Part model, mm, in its own coordinate system. A direction names the side the tool comes from. Give positions to 0.01 mm unless a question says otherwise; leave off trailing zeros. Write each loop counter-clockwise with the first axis right and the second up, starting at its lowest first coordinate (ties: lowest second). Pieces come first, ordered by that corner, then holes.
```python
from build123d import *

# Parameters (mm, degrees)
CROQUIS1_W              = 50
CROQUIS1_H              = 25
SALIENTE_EXTRUIR1_DEPTH = 20
SALIENTE_EXTRUIR2_DEPTH = 25
SALIENTE_EXTRUIR3_DEPTH = 2
CROQUIS3_W              = 40
CROQUIS3_H              = 23
CORTAR_EXTRUIR1_DEPTH   = 20
CHAFL_N1_SIZE           = 5
CHAFL_N1_SIZE2          = 5.958767963


with BuildPart() as part:
    # Croquis1 → Saliente-Extruir1 (new body)
    with BuildSketch(Plane(origin=(0, 0, 0), x_dir=(1, 0, 0), z_dir=(0, 1, 0))):
        Rectangle(CROQUIS1_W, CROQUIS1_H)
    extrude(amount=SALIENTE_EXTRUIR1_DEPTH)

    # Croquis2 → Saliente-Extruir2 (add)
    with BuildSketch(Plane.XY.offset(12.5)):
        with BuildLine():
            ThreePointArc((25, 20), (3, 42), (-19, 20))
            Line((-19, 20), (-17, 20))
            ThreePointArc((-17, 20), (3, 40), (23, 20))
            Line((23, 20), (25, 20))
        make_face()
    extrude(amount=-SALIENTE_EXTRUIR2_DEPTH)

    # Croquis2<6> → Saliente-Extruir3 (add)
    with BuildSketch(Plane.XY.offset(12.5)):
        with BuildLine():
            ThreePointArc((23, 20), (3, 40), (-17, 20))
            Line((-17, 20), (23, 20))
        make_face()
    extrude(amount=-SALIENTE_EXTRUIR3_DEPTH)

    # Croquis3 → Cortar-Extruir1 (cut)
    with BuildSketch(Plane(origin=(0, 20, 0), x_dir=(1, 0, 0), z_dir=(0, 1, 0))):
        with Locations((3, 1)):
            Rectangle(CROQUIS3_W, CROQUIS3_H)
    extrude(amount=-CORTAR_EXTRUIR1_DEPTH, mode=Mode.SUBTRACT)

    # Chaflán1
    chafl_n1_edges = [part.edges().sort_by_distance(p)[0] for p in [
        (-25, 20, 0),
    ]]
    chafl_n1_side = [part.faces().sort_by_distance(p)[0] for p in [
        (-25, 10, 0),
    ]]
    chamfer(chafl_n1_edges, length=CHAFL_N1_SIZE, length2=CHAFL_N1_SIZE2, reference=chafl_n1_side[0])


solid = part.part
```
1) 3-axis set-ups, long thin cutter, end or side, ignore diameter. For faces 5 (the face through (-21.979, 17.535, 0.175)), 6 (the face through (-17, 10, -1)): which of +Z, -Z, +X, -X, +Y, -Y reach the whole face in a straight line?
Answers follow:
face 5: +Z, -Z, -X, +Y
face 6: -Z, -Y
2) Saw through at C-C, the plane y = 12.5. Write the cut outline in (x, z), then the cut area to 3 significant figures.
Answers follow:
outline: (-25, -12.5) - (-17, -12.5) - (-17, 10.5) - (23, 10.5) - (23, -12.5) - (25, -12.5) - (25, 12.5) - (-25, 12.5) - close
area: 330 mm2
3) Saw through at B-B, the plane x = 3. Write the cut outline in (y, z).
Answers follow:
outline: (0, 10.5) - (40, 10.5) - (40, -12.5) - (42, -12.5) - (42, 12.5) - (0, 12.5) - close
4) Pin check, flat tips, straight feed: pin 1 Ø10 at (x, z) = (-8, 10) entering from +Y; pin 2 Ø2 at (x, z) = (8.5, -9) entering from -Y; pin 3 Ø1.5 at (x, y) = (8, 22) entering from -Z. Stop position of each tip, or through.
Answers follow:
pin 1: stops at y = 41.17
pin 2: stops at y = 38.91
pin 3: stops at z = 10.5
5) Wall check: L1, parallel to X at y = 12, z = 10; L2, parallel to Z at x = 8, y = 34.5; L3, parallel to X at y = 37, z = 9.5. Give the ranges that are in metal, low to high.
Answers follow:
L1: x = -25 to -17, 23 to 25
L2: z = 10.5 to 12.5
L3: x = -10.96 to -7.54, 13.54 to 16.96
6) Saw through at D-D, the plane x = -7.5. Write the cut outline in (y, z).
Answers follow:
outline: (0, 10.5) - (37.02, 10.5) - (37.02, -12.5) - (39.33, -12.5) - (39.33, 12.5) - (0, 12.5) - close
7) Two-plate mould, pull along X, no slides. Class faces 1 (the face through (-9, 0, 12)), 2 (the face through (3, 40, -1)), 3 (the face through (25, 10, 0)), 4 (the face through (23, 10, -1)): +X half, -X half, draft (parallel to the pull), parting line (faces both ways), or undercut.
Answers follow:
face 1: draft
face 2: undercut
face 3: +X half
face 4: undercut
8) Saw through at A-A, the plane z = -8.5. Write the cut outline in (x, y).
Answers follow:
outline: (-25, 0) - (-17, 0) - (-17, 20) arc R20 cw to (23, 20) - (23, 0) - (25, 0) - (25, 20) arc R22 ccw to (-19, 20) - (-19.04, 20) - (-25, 15) - close
